Geometry: see drawing. Coordinates: mm, zero at the bounding-box minimum. Coordinates: 2 decimals unless noted, no trailing zeros. Order: outer loops, then holes, each group sorted by start corner. A loop starts at its lowest first (then second) coordinate and runs counter-clockwise, first axis right, second up.
Item 1: Ray query, line 1 (Y direction, x = 30, z = 55); line 2 (Z direction, x = 19, y = 79); line 3 (Z direction, x = 25, y = 40.5). Return the intervals inside material, ascending.
Item 2: Mould query, pull axis Y, two halves, no side actions, for the marked faces 1, 2 and 3. Classes: released by +Y, released by -Y, zero draft, split by the parting line, or undercut.
Item 3: Contact query for flat-ended pins moving along their axis: P1, Ø6, axis at y = 27, z = 36.5, coming from the -X side; P2, Ø8, axis at x = 28.5, y = 34.5, coming from the -Z side; P3, Ø4, axis at x = 28, z = 65, coming from the +Y side; P4, Ø4, axis at x = 24, z = 35, coming from the +Y side. Output: stop coordinate, or through.
Item 4: Section A-A on y = 55. Return the cut outline in (x, z).
Item 5: Section C-C on x = 29. Return the cut outline in (y, z).
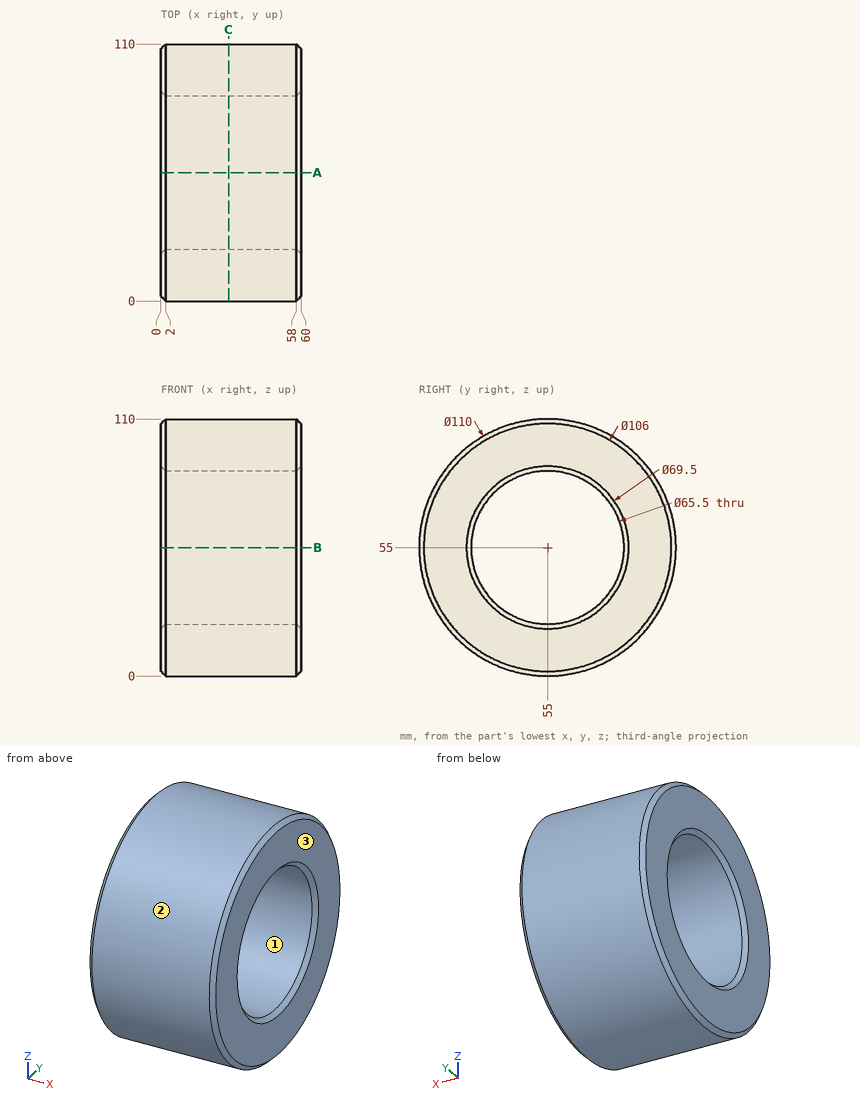
Answer list:
1. line 1: y = 0 to 22.25, 87.75 to 110
1. line 2: z = 5.51 to 32.72, 77.28 to 104.49
1. line 3: z = 1.95 to 25.63, 84.37 to 108.05
2. face 1: undercut
2. face 2: split by the parting line
2. face 3: zero draft
3. P1: stops at x = 0
3. P2: stops at z = 2.53
3. P3: stops at y = 109.42
3. P4: stops at y = 106.97
4. outline: (0, 2) - (2, 0) - (58, 0) - (60, 2) - (60, 20.25) - (58, 22.25) - (2, 22.25) - (0, 20.25) - close; (0, 89.75) - (2, 87.75) - (58, 87.75) - (60, 89.75) - (60, 108) - (58, 110) - (2, 110) - (0, 108) - close
5. outline: circle Ø110 at (55, 55); hole circle Ø65.5 at (55, 55)
